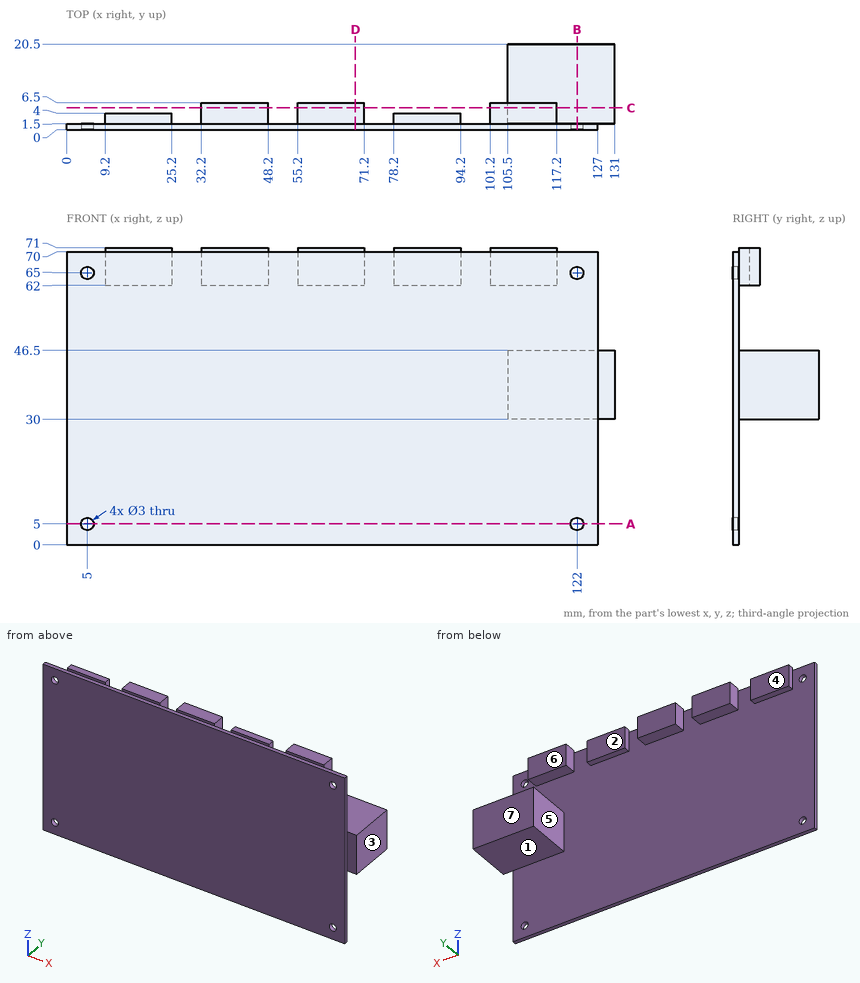
Here's the drawing with two shaded views (mm, measured from the low corner). I have some questions. A direction names the side the tool comes from. Give positions to 0.01 mm unless a question says otherwise; leave off trailing zeros. Loops run counter-clockwise (first coordinate to the right, second up) from the corner with the lowest first, then second, coordinate; pieces in that order, holes last. Notation, with made-up numbers: M 67.25,75 L 85.25,75 A23 cw 85.25,97 Z; hole C 28.5,72.5 d5. An arc over 180 degrees is marked long. One line per item, written item: value.
(1) I need wall thicknesses on line 1 (X direction, y = 0.3, z = 5); line 2 (Z direction, x = 5, y = 1.1); line 3 (Z direction, x = 114.5, y = 2.5). Which ranges of each line are inside material? Lowest first, please.
Returned:
line 1: 0 to 3.5, 6.5 to 120.5, 123.5 to 127
line 2: 0 to 3.5, 6.5 to 63.5, 66.5 to 70
line 3: 30 to 46.5, 62 to 71
(2) We'd pull the mould along X, two halves only. Please class the marked faces 1, 2 and 3: released by +X, released by -X, zero draft, split by the parting line, or undercut.
Returned:
face 1: zero draft
face 2: undercut
face 3: released by +X
(3) Suppose I cut it at D-D on x = 69. List the corners of the cut face in (y, z) for me.
Returned:
outline: M 0,0 L 1.5,0 L 1.5,62 L 6.5,62 L 6.5,71 L 1.5,71 L 1.5,70 L 0,70 Z
(4) Which directions (+Z, -Z, +X, -X, +Y, -Y) give clear straight access to the entire face, cutting with the end or side of a thin tool? Please do the marked faces 4, 5, 6 and 7.
Returned:
face 4: +Z, -Z, -X, +Y
face 5: -Z, -X, +Y
face 6: +Z, +X, -X, +Y
face 7: +Z, -Z, +X, -X, +Y
(5) Suppose I cut it at A-A on z = 5. List the corners of the cut face in (x, y) for me.
Returned:
outline: M 0,0 L 3.5,0 L 3.5,1.5 L 0,1.5 Z; M 6.5,0 L 120.5,0 L 120.5,1.5 L 6.5,1.5 Z; M 123.5,0 L 127,0 L 127,1.5 L 123.5,1.5 Z
(6) Will these pins go through, and if not, where does the flat tip stop? pin 1 (12 mm diameter, centred on y = 15.5, z = 61.5, fed in from +X) (1 decimal); pin 2 (2.5 mm diameter, centred on y = 3, z = 67.5, fed in from +X); pin 3 (4 mm diameter, centred on y = 3, z = 67, fed in from +X); pin 4 (4.5 mm diameter, centred on x = 63, z = 65.5, fed in from +Y).
Returned:
pin 1: through
pin 2: x = 117.2
pin 3: x = 127
pin 4: y = 6.5
(7) Suppose I cut it at C-C on y = 5.25. List the corners of the cut face in (x, z) for me, plus the area to 3 significant figures.
Returned:
outline: M 32.2,62 L 48.2,62 L 48.2,71 L 32.2,71 Z; M 55.2,62 L 71.2,62 L 71.2,71 L 55.2,71 Z; M 101.2,62 L 117.2,62 L 117.2,71 L 101.2,71 Z; M 105.5,30 L 131,30 L 131,46.5 L 105.5,46.5 Z
area: 853 mm^2
(8) Suppose I cut it at B-B on x = 122. List the corners of the cut face in (y, z) for me, plus the area to 4 significant figures.
Returned:
outline: M 0,0 L 1.5,0 L 1.5,3.5 L 0,3.5 Z; M 0,6.5 L 1.5,6.5 L 1.5,30 L 20.5,30 L 20.5,46.5 L 1.5,46.5 L 1.5,63.5 L 0,63.5 Z; M 0,66.5 L 1.5,66.5 L 1.5,70 L 0,70 Z
area: 409.5 mm^2
